Work out the finished part from the listing and answer in its coordinate system (mm). Round coordinates to 2 decimals unless told otherwise and drop trailing zeros. Order: outer loops, then holes, each group sorted by start corner. A loop starts at its lowest first (then second) coordinate and runs counter-clockwise, first axis right, second up. Notation, with made-up numbers: (25, 39) - (30, 39) arc R29 ccw to (30, 61) - close; hole circle Ø6 at (-20.75, -39). An arc over 180 degrees is marked (long way). Answer in a Markdown table with one row per item.
from build123d import *

# Parameters (mm, degrees)
SKETCH1_R           = 2.032
BOSS_EXTRUDE1_DEPTH = 3.175
FILLET1_R           = 3.175


with BuildPart() as part:
    # Sketch1 → Boss-Extrude1 (new body)
    with BuildSketch(Plane.XY):
        with BuildLine():
            Line((0, 114.3), (114.3, 114.3))
            Line((114.3, 114.3), (88.9, 86.353963576))
            ThreePointArc((88.9, 86.353963576), (69.85, 101.6), (50.8, 86.353963576))
            Line((50.8, 86.353963576), (50.8, 0))
            Line((50.8, 0), (0, 0))
            Line((0, 0), (0, 63.5))
            Line((0, 63.5), (0, 114.3))
        make_face()
        with Locations((9.525, 14.869716291)):
            Circle(SKETCH1_R, mode=Mode.SUBTRACT)
        with Locations((41.275, 14.869716291)):
            Circle(SKETCH1_R, mode=Mode.SUBTRACT)
        with Locations((25.4, 6.35)):
            Circle(SKETCH1_R, mode=Mode.SUBTRACT)
        with Locations((25.4, 25.4)):
            Circle(SKETCH1_R, mode=Mode.SUBTRACT)
        with Locations((12.432008635, 39.354701715)):
            Circle(SKETCH1_R, mode=Mode.SUBTRACT)
    extrude(amount=BOSS_EXTRUDE1_DEPTH)

    # Fillet1
    fillet1_edges = [part.edges().sort_by_distance(p)[0] for p in [
        (0, 114.3, 1.5875),
        (114.3, 114.3, 1.5875),
        (88.9, 86.353963576, 1.5875),
        (50.8, 0, 1.5875),
        (0, 0, 1.5875),
    ]]
    fillet(fillet1_edges, radius=FILLET1_R)


solid = part.part
1) Find section A-A, the plane y = 6.35. Give the vertices of the cut face in (x, z) (3 decimals), then the cut area to 3 significant figures.
Filled in:
| item | result |
|---|---|
| outline | (0, 0) - (23.368, 0) - (23.368, 3.175) - (0, 3.175) - close; (27.432, 0) - (50.8, 0) - (50.8, 3.175) - (27.432, 3.175) - close |
| area | 148 mm^2 |
2) Find section C-C, the plane z = 2.5. Give the vertices of the cut face in (x, y) (3 decimals).
Filled in:
| item | result |
|---|---|
| outline | (0, 3.175) arc R3.175 ccw to (3.175, 0) - (47.625, 0) arc R3.175 ccw to (50.8, 3.175) - (50.8, 86.354) arc R19.525 cw to (87.25, 90.932) arc R3.175 ccw to (92.429, 90.237) - (109.473, 108.99) arc R3.175 ccw to (107.124, 114.3) - (3.175, 114.3) arc R3.175 ccw to (0, 111.125) - close; hole circle Ø4.064 at (9.525, 14.87); hole circle Ø4.064 at (12.432, 39.355); hole circle Ø4.064 at (25.4, 6.35); hole circle Ø4.064 at (25.4, 25.4); hole circle Ø4.064 at (41.275, 14.87) |
3) Find section D-D, the plane y = 54. Give the vertices of the cut face in (x, z) (3 decimals), then the cut area to 3 significant figures.
Filled in:
| item | result |
|---|---|
| outline | (0, 0) - (50.8, 0) - (50.8, 3.175) - (0, 3.175) - close |
| area | 161 mm^2 |
4) The mould has two halves that part along X. Classify faces 1 (the face through (50.8, 45, 2)), 2 (the face through (31, 71, 3.175)), 3 (the face through (9.085, 12.886, 1.565)): released by +X, released by -X, zero draft, split by the parting line, or undercut.
Filled in:
| item | result |
|---|---|
| face 1 | released by +X |
| face 2 | zero draft |
| face 3 | undercut |
5) Find the intervals of material crossed by probe 1 along Y at (x, z) = (25.4, 2.2); probe 2 along X at (y, z) = (13.5, 0.3); probe 3 along X at (y, z) = (33.5, 2.5), in increasing order. Write a range as from..to.
Filled in:
| item | result |
|---|---|
| probe 1 | y = 0..4.32, 8.38..23.37, 27.43..114.3 |
| probe 2 | x = 0..8.02, 11.03..39.77, 42.78..50.8 |
| probe 3 | x = 0..50.8 |
6) Find section B-B, the plane x = 25.4. Give the vertices of the cut face in (y, z) (3 decimals), then the cut area to 3 significant figures.
Filled in:
| item | result |
|---|---|
| outline | (0, 0) - (4.318, 0) - (4.318, 3.175) - (0, 3.175) - close; (8.382, 0) - (23.368, 0) - (23.368, 3.175) - (8.382, 3.175) - close; (27.432, 0) - (114.3, 0) - (114.3, 3.175) - (27.432, 3.175) - close |
| area | 337 mm^2 |
